Design review of the part built by this model. Coordinates are the model's own, in mm. A direction names the side the tool comes from. Give positions to 0.01 mm unless a question says otherwise; leave off trailing zeros. Loops run counter-clockwise (first coordinate to the right, second up) from the corner with the lowest first, then second, coordinate; pieces in that order, holes last. Notation, with made-up numbers: (-34, 82) -> (-17, 82) arc R23 cw to (-17, 107) -> close; hole circle Ø2 at (-21, -32). An arc over 180 degrees is marked (long way). Answer in a Markdown table with one row per item. Add a question column.
(1) For pin 1 (2 mm diameter, centred on x = 1.5, z = 4.5, fed in from -Y); pin 2 (0.8 mm diameter, centred on x = 3, z = 27, fed in from -Y); pin 3 (0.5 mm diameter, centred on y = 1.5, z = 27, fed in from +X), all flat-tipped, find the tip position at first contact; note any pin that passes through.
(2) Consider section A-A on x = 0. Write out the cut boundary in (y, z), then the cut area to 3 significant figures.
(3) Consider section B-B on y = 3.75. Write out the cut boundary in (x, z).
(4) Draft analysis for pull direction X (two halves, no side actions). For faces 5 (the cylindrical face through (0, -2, 14)), 6 (the flat face through (0, 0, 26.4)), 7 (the flat face through (2, -1, 1.2)), 8 (the flat face through (0.5, -1, 27)), state which applies: +X half, -X half, draft (parallel to the pull), parting line (faces both ways), or undercut.
(5) Consider section D-D on x = 2.25. Write out the cut boundary in (y, z), then the cut area to 3 significant figures.
(6) Consider section C-C on y = 0. Write out the cut boundary in (x, z), then the cut area to 3 significant figures.
(7) For line 1 (Z direction, x = -2, y = 2.5); line 2 (Z direction, x = 3.5, y = -2.5); line 3 (Z direction, x = -1, y = 0), list the stretches that pass through material, from the lowest coordinate up.
(8) For faces 1 (the cylindrical face through (4.054, 1.277, 0.592)), 2 (the flat face through (-0.1, 0.5, 0.5)), 3 (the flat face through (2, -1, 26.2)), 4 (the flat face through (3, 0.5, 27)), list the 3-axis set-ups (+Z, -Z, +X, -X, +Y, -Y) from which the entire face can be reached by the end or side of a thin tool; tool diameter is ignored.
from build123d import *

# Parameters (mm, degrees)
SKETCH_1_R          = 4.25
EXTRUDE_1_DEPTH     = 1.2
SKETCH_2_R          = 2
EXTRUDE_2_DEPTH     = 25
SKETCH_3_R          = 4.75
EXTRUDE_3_DEPTH     = 1.2
CUT_EXTRUDE_START   = -1
CUT_EXTRUDE_1_DEPTH = 1
CUT_EXTRUDE_2_DEPTH = 1


with BuildPart() as part:
    # 草图1 → 凸台-拉伸1 (new body)
    with BuildSketch(Plane.XY):
        Circle(SKETCH_1_R)
    extrude(amount=EXTRUDE_1_DEPTH)

    # 草图2 → 凸台-拉伸2 (add)
    with BuildSketch(Plane.XY.offset(1.2)):
        Circle(SKETCH_2_R)
    extrude(amount=EXTRUDE_2_DEPTH)

    # 草图3 → 凸台-拉伸3 (add)
    with BuildSketch(Plane.XY.offset(26.2)):
        Circle(SKETCH_3_R)
    extrude(amount=EXTRUDE_3_DEPTH)

    # 草图4 → 切除-拉伸1 (cut)
    with BuildSketch(Plane.XY.offset(27.4).offset(CUT_EXTRUDE_START)):
        with BuildLine():
            Line((-0.5, 2), (-0.5, 0.5))
            Line((-0.5, 0.5), (-4.723610907, 0.5))
            ThreePointArc((-4.723610907, 0.5), (-4.75, 0), (-4.723610907, -0.5))
            Line((-4.723610907, -0.5), (-0.5, -0.5))
            Line((-0.5, -0.5), (-0.5, -2))
            Line((-0.5, -2), (0.5, -2))
            Line((0.5, -2), (0.5, -0.5))
            Line((0.5, -0.5), (4.723610907, -0.5))
            ThreePointArc((4.723610907, -0.5), (4.75, 0), (4.723610907, 0.5))
            Line((4.723610907, 0.5), (0.5, 0.5))
            Line((0.5, 0.5), (0.5, 2))
            Line((0.5, 2), (-0.5, 2))
        make_face()
    extrude(amount=CUT_EXTRUDE_1_DEPTH, mode=Mode.SUBTRACT)

    # 草图5 → 切除-拉伸2 (cut)
    with BuildSketch(Plane(origin=(0, 0, 0), x_dir=(-1, 0, 0), z_dir=(0, 0, -1))):
        with BuildLine():
            Line((-4.723610907, -0.5), (4.723610907, -0.5))
            ThreePointArc((4.723610907, -0.5), (4.75, 0), (4.723610907, 0.5))
            Line((4.723610907, 0.5), (-4.723610907, 0.5))
            ThreePointArc((-4.723610907, 0.5), (-4.75, 0), (-4.723610907, -0.5))
        make_face()
    extrude(amount=-CUT_EXTRUDE_2_DEPTH, mode=Mode.SUBTRACT)


solid = part.part
Values follow:
| question | item | result |
|---|---|---|
| 1 | pin 1 | y = -1.94 |
| 1 | pin 2 | y = -3.98 |
| 1 | pin 3 | x = 4.58 |
| 2 | outline | (-4.75, 26.2) -> (-2, 26.2) -> (-2, 1.2) -> (-4.25, 1.2) -> (-4.25, 0) -> (-0.5, 0) -> (-0.5, 1) -> (0.5, 1) -> (0.5, 0) -> (4.25, 0) -> (4.25, 1.2) -> (2, 1.2) -> (2, 26.2) -> (4.75, 26.2) -> (4.75, 27.4) -> (2, 27.4) -> (2, 26.4) -> (-2, 26.4) -> (-2, 27.4) -> (-4.75, 27.4) -> close |
| 2 | area | 117 mm2 |
| 3 | outline | (-2.92, 26.2) -> (2.92, 26.2) -> (2.92, 27.4) -> (-2.92, 27.4) -> close; (-2, 0) -> (2, 0) -> (2, 1.2) -> (-2, 1.2) -> close |
| 4 | face 5 | parting line |
| 4 | face 6 | undercut |
| 4 | face 7 | draft |
| 4 | face 8 | undercut |
| 5 | outline | (-4.18, 26.2) -> (4.18, 26.2) -> (4.18, 27.4) -> (0.5, 27.4) -> (0.5, 26.4) -> (-0.5, 26.4) -> (-0.5, 27.4) -> (-4.18, 27.4) -> close; (-3.61, 0) -> (-0.5, 0) -> (-0.5, 1) -> (0.5, 1) -> (0.5, 0) -> (3.61, 0) -> (3.61, 1.2) -> (-3.61, 1.2) -> close |
| 5 | area | 16.7 mm2 |
| 6 | outline | (-4.75, 26.2) -> (-2, 26.2) -> (-2, 1.2) -> (-4.25, 1.2) -> (-4.25, 1) -> (4.25, 1) -> (4.25, 1.2) -> (2, 1.2) -> (2, 26.2) -> (4.75, 26.2) -> (4.75, 26.4) -> (-4.75, 26.4) -> close |
| 6 | area | 104 mm2 |
| 7 | line 1 | 0 to 1.2, 26.2 to 27.4 |
| 7 | line 2 | 26.2 to 27.4 |
| 7 | line 3 | 1 to 26.4 |
| 8 | face 1 | -Z |
| 8 | face 2 | -Z, +X, -X |
| 8 | face 3 | none |
| 8 | face 4 | +Z, +X, -X |
